from build123d import *

# Parameters (mm, degrees)
SCALE1_SCALE = 0.85770751


with BuildPart() as part:
    # Sketch1 → Revolve25 (revolve)
    with BuildSketch(Plane.XY):
        with BuildLine():
            Line((-5.582614804, -1.992146118), (-5.6, 0))
            Line((-5.6, 0), (-7.4, 0))
            Line((-7.4, 0), (-7.4, -2))
            Line((-7.4, -2), (-6.482580535, -2))
            Line((-6.482580535, -2), (-6.325496915, -20))
            Line((-6.325496915, -20), (-3.834959356, -35.724635285))
            ThreePointArc((-3.834959356, -35.724635285), (-2.521652597, -38.069713242), (0, -39))
            Line((0, -39), (0, -38.1))
            ThreePointArc((0, -38.1), (-1.937149354, -37.385347873), (-2.946039849, -35.583844266))
            Line((-2.946039849, -35.583844266), (-5.426114828, -19.925267112))
            Line((-5.426114828, -19.925267112), (-5.582614804, -1.992146118))
        make_face()
    revolve(axis=Axis((0, 0, 0), (0, -1, 0)))


with BuildPart() as part_1:
    # Scale1: scaled about (0, -16.444791582, 0)
    add(part.part.scale(SCALE1_SCALE).moved(Location((0, -2.339970344, 0))))


solid = part_1.part
Build history of the part. All positions in model axes, mm. A direction names the side the tool comes from. Round coordinates to 2 decimals unless told otherwise and drop trailing zeros. Loops run counter-clockwise (first coordinate to the right, second up) from the corner with the lowest first, then second, coordinate; pieces in that order, holes last. Notation, with made-up numbers: (66.25, 30) -> (117.25, 30) arc R11 ccw to (117.25, 45) -> close; hole circle Ø7 at (27.25, -35.5). An arc over 180 degrees is marked (long way). Use CSV: the item, a comma, the result in double quotes. Start each with the question number.
Q1. Drill centre lines: L1, parallel to Z at x = -0.5, y = -17; L2, parallel to Y at x = -2.75, z = -5; L3, parallel to Z at x = -3, y = -24.5. Where is each one in solid material? Low to high.
Q2. Which spindle directions (+Z, -Z, +X, -X, +Y, -Y) get a long thin tool onto all of the face, cutting with end or side? Do faces 4 (the face through (-1, -2.34, -5)), 5 (the face through (1.19, -11.88, 5.36)). Say none if no direction does.
Q3. Saw through at B-B on y = -24. Give the cut face in (x, z).
Q4. Flat gauge pins, fed straight in: pin 1 Ø4 at (y, z) = (-29.5, 0.5) entering from +X; pin 2 Ø1 at (y, z) = (-12, 2.5) entering from +X. Where does each tip first touch, or does it go through?
Q5. Mould opens along X. For faces 1 (the face through (0, -4.055, 6)), 2 (the face through (-3.412, -3.21, -5.352)), 3 (the face through (0.78, -26.05, 3.52)) say: +X half, -X half, draft (parallel to the pull), parting line (faces both ways), or undercut.
Q6. Saw through at A-A on y = -29. Give the cut face in (x, z).
Solutions:
1,L1,"z = -5.42 to -4.65, 4.65 to 5.42"
1,L2,"y = -4.06 to -2.34"
1,L3,"z = -3.53 to -2.41, 2.41 to 3.53"
2,face 4,"+Z, -Z, +X, -X, +Y"
2,face 5,"-Y"
3,outline,"circle Ø9.42 at (0, 0); hole circle Ø7.86 at (0, 0)"
4,pin 1,"stops at x = 4.15"
4,pin 2,"stops at x = 5.11"
5,face 1,"draft"
5,face 2,"parting line"
5,face 3,"undercut"
6,outline,"circle Ø7.84 at (0, 0); hole circle Ø6.28 at (0, 0)"
